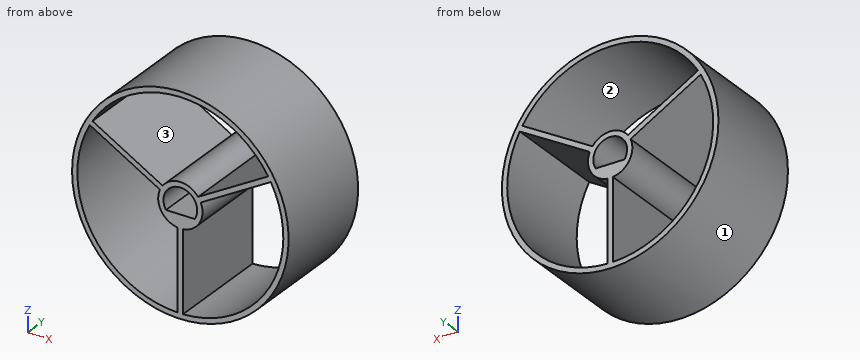
Autodesk Inventor part; units mm, degrees
ref_plane "YZ Plane" through (0, 0, 0) normal (1, 0, 0) x (0, 1, 0)
ref_plane "XZ Plane" through (0, 0, 0) normal (0, 1, 0) x (-1, 0, 0)
ref_plane "XY Plane" through (0, 0, 0) normal (0, 0, 1) x (1, 0, 0)
sketch "Sketch1" plane through (0, 0, 0) normal (0, 1, 0) x (-1, 0, 0)
  circle A0 centre (0, 0) radius 61.5
  dimension "d0" = 123
extrude "Extrusion1" add sketch "Sketch1" along normal blind 60
thread "Thread1"
sketch "Sketch2" plane through (0, 60, 0) normal (0, 1, 0) x (1, 0, 0)
  arc A0 (-8.1881, 5) -> (8.1881, 5) centre (0, 0) ccw
  line L0 (-8.1881, 5) -> (8.1881, 5)
  dimension "d5" = 19.188
  dimension "d6" = 5
extrude "Extrusion2" cut sketch "Sketch2" against normal up to surface (60 mm away)
sketch "Sketch3" plane through (0, 60, 0) normal (0, 1, 0) x (1, 0, 0)
  line L0 (-8.1881, 5) -> (8.1881, 5)
  arc A0 (-8.1881, 5) -> (8.1881, 5) centre (0, 0) ccw
  circle A1 centre (0, 0) radius 61.5
  line L1 (-1.5, 58.4808) -> (-1.5, 12.5044)
  line L2 (1.5, 58.4808) -> (1.5, 12.5044)
  line L3 (-49.8958, -30.5394) -> (-10.0791, -7.5512)
  line L4 (-51.3958, -27.9413) -> (-11.5791, -4.9531)
  line L5 (51.3958, -27.9413) -> (11.5791, -4.9531)
  line L6 (49.8958, -30.5394) -> (10.0791, -7.5512)
  arc A2 (11.5791, -4.9531) -> (1.5, 12.5044) centre (0, 0) ccw
  arc A3 (-1.5, 12.5044) -> (-11.5791, -4.9531) centre (0, 0) ccw
  arc A4 (-10.0791, -7.5512) -> (10.0791, -7.5512) centre (0, 0) ccw
  arc A5 (-49.8958, -30.5394) -> (49.8958, -30.5394) centre (0, 0) ccw
  arc A6 (51.3958, -27.9413) -> (1.5, 58.4808) centre (0, 0) ccw
  arc A7 (-1.5, 58.4808) -> (-51.3958, -27.9413) centre (0, 0) ccw
  dimension "d11" = 3
  dimension "d14" = 360
extrude "Extrusion3" cut sketch "Sketch3" against normal through all contours L1 A3 L4 A7 | A6 L5 A2 L2 | L3 A4 L6 A5
properties part number "Wheel_Actual-wheel-ENES100OSVproject-spencermical-3-3-16_thursday-1-17am-freshmanyear-springsemester"
Model file for the job. Use its own axes, mm. Face numbers are marked on the shaded views. Coordinates: 2 decimals unless noted, no trailing zeros. Order: outer loops, then holes, each group sorted by start corner. A loop starts at its lowest first (then second) coordinate and runs counter-clockwise, first axis right, second up. Notation, with made-up numbers: (49, 27.5) -> (54, 27.5) arc R27 ccw to (54, 63.5) -> close; hole circle Ø1 at (-39, -39.75). An arc over 180 degrees is marked (long way). Return JSON: item names as keys, results as strings.
Item 1: Wall check: line 1 along Z through (x, y) = (0, 40); line 2 along X through (y, z) = (47.5, 23); line 3 along X through (y, z) = (26, -35.5). Give the ranges that are in metal, low to high. Write a range as from..to.
Model answer:
{"line 1": "z = -61.5..-5, 9.59..12.59, 58.5..61.5", "line 2": "x = -57.04..-53.79, -42.84..-36.84, 36.84..42.84, 53.79..57.04", "line 3": "x = -50.22..-46.5, -1.5..1.5, 46.5..50.22"}
Item 2: Slice it at C-C (y = 45). Write the cut outline in (x, z).
Model answer:
{"outline": "circle Ø123 at (0, 0); hole (-51.4, 27.94) arc R58.5 ccw to (-1.5, -58.48) -> (-1.5, -12.5) arc R12.59 cw to (-11.58, 4.95) -> close; hole (-49.9, 30.54) -> (-10.08, 7.55) arc R12.59 cw to (10.08, 7.55) -> (49.9, 30.54) arc R58.5 ccw to start; hole (-8.19, -5) -> (8.19, -5) arc R9.59 ccw (long way) to start; hole (1.5, -58.48) arc R58.5 ccw to (51.4, 27.94) -> (11.58, 4.95) arc R12.59 cw to (1.5, -12.5) -> close"}
Item 3: Slice it at D-D (z = -43). Write the cut outline in (x, y).
Model answer:
{"outline": "(-43.97, 0) -> (-39.66, 0) -> (-39.66, 60) -> (-43.97, 60) -> close; (-1.5, 0) -> (1.5, 0) -> (1.5, 60) -> (-1.5, 60) -> close; (39.66, 0) -> (43.97, 0) -> (43.97, 60) -> (39.66, 60) -> close"}
Item 4: Slice it at B-B (z = 0). Write the cut outline in (x, y).
Model answer:
{"outline": "(-61.5, 0) -> (-58.5, 0) -> (-58.5, 60) -> (-61.5, 60) -> close; (-12.59, 0) -> (-9.59, 0) -> (-9.59, 60) -> (-12.59, 60) -> close; (9.59, 0) -> (12.59, 0) -> (12.59, 60) -> (9.59, 60) -> close; (58.5, 0) -> (61.5, 0) -> (61.5, 60) -> (58.5, 60) -> close"}
Item 5: Pin check, flat tips, straight feed: P1, Ø22, axis at x = 0, z = 0, coming from the +Y side; P2, Ø12, axis at y = 28.5, z = 7, coming from the -X side; P3, Ø18, axis at x = -2.5, y = 17.5, coming from the +Z side; P4, Ø1, axis at x = -17, y = 29.5, coming from the +Z side. Stop position of each tip, or through.
Model answer:
{"P1": "stops at y = 60", "P2": "stops at x = -61.49", "P3": "stops at z = 61.5", "P4": "stops at z = 59.25"}
Item 6: Slice it at A-A (x = 0). Write the cut outline in (y, z), then the cut area to 3 significant figures.
Model answer:
{"outline": "(0, -61.5) -> (60, -61.5) -> (60, -5) -> (0, -5) -> close; (0, 9.59) -> (60, 9.59) -> (60, 12.59) -> (0, 12.59) -> close; (0, 58.5) -> (60, 58.5) -> (60, 61.5) -> (0, 61.5) -> close", "area": "3,750 mm²"}
Item 7: Mould opens along X. For the marked faces 1, 2 and 3 say: pulls with the +X half, pulls with the -X half, needs draft (parallel to the pull), parting line crosses it, or undercut.
Model answer:
{"face 1": "parting line crosses it", "face 2": "undercut", "face 3": "undercut"}
